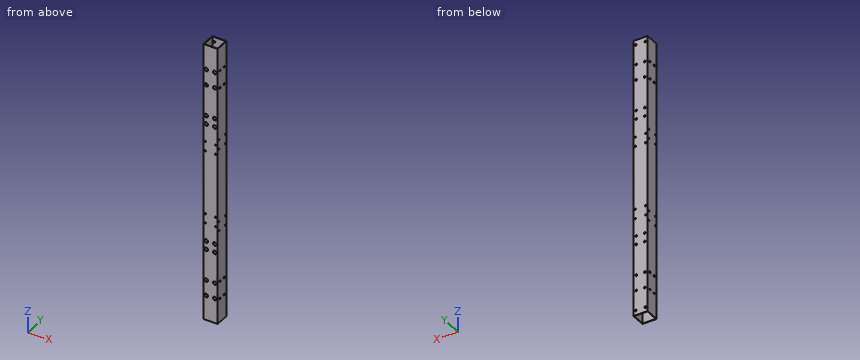
```python
from build123d import *

# Parameters (mm, degrees)
SKETCH_1_W               = 30
SKETCH_1_H               = 30
SKETCH_1_W_2             = 27.6
SKETCH_1_H_2             = 27.6
EXTRUDE_1_DEPTH          = 295
SKETCH_2_R               = 2.025
CUT_EXTRUDE_1_DEPTH      = 35
SKETCH_3_R               = 3.8
CUT_EXTRUDE_2_DEPTH      = 5
SKETCH_4_R               = 2.025
CUT_EXTRUDE_3_DEPTH      = 5
SKETCH_5_R               = 1.525
CUT_EXTRUDE_4_DEPTH      = 50
SKETCH_6_R               = 2.025
CUT_EXTRUDE_5_DEPTH      = 30
SKETCH_7_R               = 2.025
CUT_EXTRUDE_6_DEPTH      = 90
SKETCH_8_R               = 3.9
CUT_EXTRUDE_7_DEPTH      = 10
SKETCH_9_R               = 1.525
CUT_EXTRUDE_8_DEPTH      = 50
MIRROR_8_COPY_1_SKETCH_R = 1.525
MIRROR_8_COPY_1_DEPTH    = 50


with BuildPart() as part:
    # 草图1 → 凸台-拉伸1 (new body, symmetric)
    with BuildSketch(Plane.XY):
        Rectangle(SKETCH_1_W, SKETCH_1_H)
        Rectangle(SKETCH_1_W_2, SKETCH_1_H_2, mode=Mode.SUBTRACT)
    extrude(amount=EXTRUDE_1_DEPTH, both=True)

    # 草图2 → 切除-拉伸1 (cut, symmetric)
    with BuildSketch(Plane.XZ.offset(15)):
        with Locations((-9, 209.5)):
            Circle(SKETCH_2_R)
        with Locations((9, 209.5)):
            Circle(SKETCH_2_R)
        with Locations((-9, 242.5)):
            Circle(SKETCH_2_R)
        with Locations((9, 242.5)):
            Circle(SKETCH_2_R)
    cut_extrude_1 = extrude(amount=CUT_EXTRUDE_1_DEPTH, both=True, mode=Mode.SUBTRACT)

    # 镜向1: 切除-拉伸1 across plane
    add(cut_extrude_1.mirror(Plane.XY), mode=Mode.SUBTRACT)

    # 草图3 → 切除-拉伸2 (cut, symmetric)
    with BuildSketch(Plane.XZ.offset(15)):
        with Locations((9, 242.5)):
            Circle(SKETCH_3_R)
        with Locations((9, 209.5)):
            Circle(SKETCH_3_R)
        with Locations((-9, 242.5)):
            Circle(SKETCH_3_R)
        with Locations((-9, 209.5)):
            Circle(SKETCH_3_R)
    cut_extrude_2 = extrude(amount=CUT_EXTRUDE_2_DEPTH, both=True, mode=Mode.SUBTRACT)

    # 镜向2: 切除-拉伸2 across plane
    add(cut_extrude_2.mirror(Plane.XY), mode=Mode.SUBTRACT)

    # 草图4 → 切除-拉伸3 (cut, symmetric)
    with BuildSketch(Plane.XZ.offset(-13.8)):
        with Locations((-10, 285)):
            Circle(SKETCH_4_R)
        with Locations((10, 285)):
            Circle(SKETCH_4_R)
    cut_extrude_3 = extrude(amount=CUT_EXTRUDE_3_DEPTH, both=True, mode=Mode.SUBTRACT)

    # 镜向3: 切除-拉伸3 across plane
    add(cut_extrude_3.mirror(Plane.XY), mode=Mode.SUBTRACT)

    # 草图5 → 切除-拉伸4 (cut)
    with BuildSketch(Plane.XZ.offset(15)):
        with Locations((10.8, 67.5)):
            Circle(SKETCH_5_R)
        with Locations((10.8, 87.5)):
            Circle(SKETCH_5_R)
        with Locations((10.8, -87.5)):
            Circle(SKETCH_5_R)
        with Locations((10.8, -67.5)):
            Circle(SKETCH_5_R)
    cut_extrude_4 = extrude(amount=-CUT_EXTRUDE_4_DEPTH, mode=Mode.SUBTRACT)

    # 镜向4: 切除-拉伸4 across plane
    add(cut_extrude_4.mirror(Plane(origin=(0, 0, 0), x_dir=(0, 0, 1), z_dir=(1, 0, 0))), mode=Mode.SUBTRACT)

    # 草图6 → 切除-拉伸5 (cut)
    with BuildSketch(Plane.ZY.offset(15)):
        with Locations((244.5, 7)):
            Circle(SKETCH_6_R)
        with Locations((207.5, 7)):
            Circle(SKETCH_6_R)
        with Locations((207.5, -7)):
            Circle(SKETCH_6_R)
        with Locations((244.5, -7)):
            Circle(SKETCH_6_R)
        with Locations((-244.5, -7)):
            Circle(SKETCH_6_R)
        with Locations((-207.5, -7)):
            Circle(SKETCH_6_R)
        with Locations((-207.5, 7)):
            Circle(SKETCH_6_R)
        with Locations((-244.5, 7)):
            Circle(SKETCH_6_R)
    extrude(amount=-CUT_EXTRUDE_5_DEPTH, mode=Mode.SUBTRACT)

    # 草图7 → 切除-拉伸6 (cut)
    with BuildSketch(Plane.XZ.offset(15)):
        with Locations((-9, 143.5)):
            Circle(SKETCH_7_R)
        with Locations((-9, 125.5)):
            Circle(SKETCH_7_R)
        with Locations((9, 125.5)):
            Circle(SKETCH_7_R)
        with Locations((9, 143.5)):
            Circle(SKETCH_7_R)
    cut_extrude_6 = extrude(amount=-CUT_EXTRUDE_6_DEPTH, mode=Mode.SUBTRACT)

    # 镜向5: 切除-拉伸6 across plane
    add(cut_extrude_6.mirror(Plane.XY), mode=Mode.SUBTRACT)

    # 草图8 → 切除-拉伸7 (cut)
    with BuildSketch(Plane.XZ.offset(15)):
        with Locations((-9, -125.5)):
            Circle(SKETCH_8_R)
        with Locations((-9, -143.5)):
            Circle(SKETCH_8_R)
        with Locations((9, -143.5)):
            Circle(SKETCH_8_R)
        with Locations((9, -125.5)):
            Circle(SKETCH_8_R)
    cut_extrude_7 = extrude(amount=-CUT_EXTRUDE_7_DEPTH, mode=Mode.SUBTRACT)

    # 镜向6: 切除-拉伸7 across plane
    add(cut_extrude_7.mirror(Plane.XY), mode=Mode.SUBTRACT)

    # 草图9 → 切除-拉伸8 (cut)
    with BuildSketch(Plane.ZY.offset(15)):
        with Locations((97.5, -10.8)):
            Circle(SKETCH_9_R)
        with Locations((77.5, -10.8)):
            Circle(SKETCH_9_R)
    cut_extrude_8 = extrude(amount=-CUT_EXTRUDE_8_DEPTH, mode=Mode.SUBTRACT)

    # 镜向7: 切除-拉伸8 across plane
    add(cut_extrude_8.mirror(Plane.XY), mode=Mode.SUBTRACT)

    # 镜向8: 切除-拉伸8 across plane
    add(cut_extrude_8.mirror(Plane.ZX), mode=Mode.SUBTRACT)

    # 镜向8 copy 1 sketch → 镜向8 copy 1 (cut)
    with BuildSketch(Plane(origin=(-15, 0, 0), x_dir=(0, 0, -1), z_dir=(-1, 0, 0))):
        with Locations((97.5, -10.8)):
            Circle(MIRROR_8_COPY_1_SKETCH_R)
        with Locations((77.5, -10.8)):
            Circle(MIRROR_8_COPY_1_SKETCH_R)
    extrude(amount=-MIRROR_8_COPY_1_DEPTH, mode=Mode.SUBTRACT)


solid = part.part
```
Check sheet for the modelled part. Datum: model origin and axes. Units: mm. Coordinates: 2 decimals unless noted, no trailing zeros. Order: outer loops, then holes, each group sorted by start corner. A loop starts at its lowest first (then second) coordinate and runs counter-clockwise, first axis right, second up. Notation, with made-up numbers: M 63.5,83.25 L 81.5,83.25 A17 ccw 81.5,94.25 Z; hole C -4,84 d11. An arc over 180 degrees is marked long. Write each question's results on one line, items separated by ' | '. Start each with the question number.
1. Cross-section at A-A on z = -25. Record the cut outline in (x, y), and give its area (3 significant figures).
2. Go/stop test with flat-tipped pins: P1, Ø7, axis at x = 9, z = -242.5, coming from the -Y side; P2, Ø4, axis at x = -11.5, y = -3.5, coming from the -Z side. Record where each tip stops, or that it passes through.
3. Material ranges on probe 1 along X at (y, z) = (14.45, -285) (3 decimals); probe 2 along Y at (x, z) = (-14.45, -97.5) (3 decimals); probe 3 along Y at (x, z) = (-11.25, 12.5), recorded low to high.
Checks:
1) outline: M -15,-15 L 15,-15 L 15,15 L -15,15 Z; hole M -13.8,-13.8 L 13.8,-13.8 L 13.8,13.8 L -13.8,13.8 Z | area: 138 mm²
2) P1: stops at y = 13.8 | P2: passes through
3) probe 1: x = -15 to -12.025, -7.975 to 7.975, 12.025 to 15 | probe 2: y = -15 to -12.325, -9.275 to 9.275, 12.325 to 15 | probe 3: y = -15 to -13.8, 13.8 to 15
